```python
from build123d import *

# Parameters (mm, degrees)
F0_R     = 2
F1_DEPTH = 15
F2_W     = 15
F2_H     = 5
F3_DEPTH = 25.4


# Not quite as in the source:
# - a feature names something its author has since deleted; it is built from what else it names


with BuildPart() as f1:
    # F0 (on Top) → F1 (new body)
    with BuildSketch(Plane.XY):
        Polygon((-4, 0), (0, 0), (0, 15), (3, 15), (3, 0), (6, 0), (6, 25), (-4, 25), align=None)
        with Locations((1, 20)):
            Circle(F0_R, mode=Mode.SUBTRACT)
    extrude(amount=F1_DEPTH)

    # F2 (on face) → F3 (cut)
    with BuildSketch(Plane.YZ.offset(6)):
        with Locations((17.5, 7.5)):
            Rectangle(F2_W, F2_H)
    extrude(amount=-F3_DEPTH, mode=Mode.SUBTRACT)


solid = f1.part
```
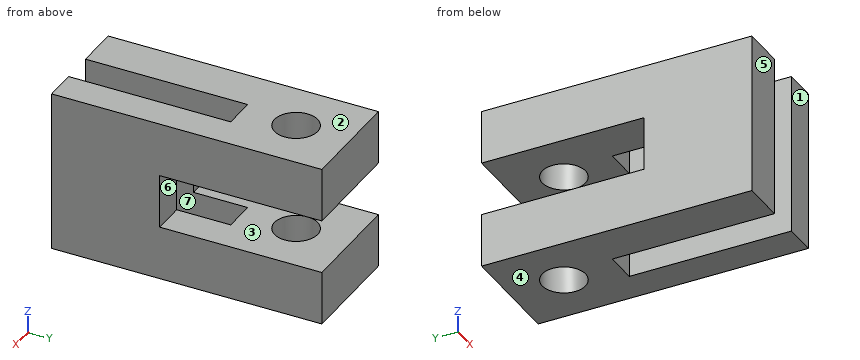
Read the model definition and answer for the solid it produces. Units are mm, in the model's axes. Face numbers are marked on the shaded views. A direction names the side the tool comes from. Give positions to 0.01 mm unless a question says otherwise; leave off trailing zeros. Order: outer loops, then holes, each group sorted by start corner. A loop starts at its lowest first (then second) coordinate and runs counter-clockwise, first axis right, second up.
(1) Find section C-C (z = 12). Give the vertices of the cut face in (x, y).
(2) Find section D-D (y = 20). Give the vertices of the cut face in (x, z).
(3) For a pull along Z with two mould halves and no side action, classify the marked faces 1, 2, 3 and 4 as released by +Z, released by -Z, zero draft, split by the parting line, or undercut.
(4) Find section B-B (y = 2.5). Give the vertices of the cut face in (x, z), plus the area to 3 significant figures.
(5) Find section A-A (x = 1). Give the vertices of the cut face in (y, z).
(6) Given pin 1 (0.9 mm diameter, centred on x = 1, z = 12.5, fed in from -Y); pin 2 (2 mm diameter, centred on x = -2, z = 8.5, fed in from +Y), each flat-ended and moving along its own axis, determine where each tip first touches the part or whether it passes through.
(7) For the marked faces 5, 6 and 7, determine the directions among +Z, -Z, +X, -X, +Y, -Y from which every point of the face is accessible in a straight line to the end or side of a thin tool.
(8) Straight lines are drawn through the part: L1, parallel to Z at x = 2.75, y = 16; L2, parallel to Y at x = 1, z = 11.1; L3, parallel to X at y = 20, z = 13.2. For each, find the intervals that lie inside material, in ascending order.
Result sheet:
1. outline: (-4, 0) - (0, 0) - (0, 15) - (3, 15) - (3, 0) - (6, 0) - (6, 25) - (-4, 25) - close; hole circle Ø4 at (1, 20)
2. outline: (-4, 0) - (-1, 0) - (-1, 5) - (-4, 5) - close; (-4, 10) - (-1, 10) - (-1, 15) - (-4, 15) - close; (3, 0) - (6, 0) - (6, 5) - (3, 5) - close; (3, 10) - (6, 10) - (6, 15) - (3, 15) - close
3. face 1: zero draft
3. face 2: released by +Z
3. face 3: undercut
3. face 4: released by -Z
4. outline: (-4, 0) - (0, 0) - (0, 15) - (-4, 15) - close; (3, 0) - (6, 0) - (6, 15) - (3, 15) - close
4. area: 105 mm2
5. outline: (15, 0) - (18, 0) - (18, 5) - (15, 5) - close; (15, 10) - (18, 10) - (18, 15) - (15, 15) - close; (22, 0) - (25, 0) - (25, 5) - (22, 5) - close; (22, 10) - (25, 10) - (25, 15) - (22, 15) - close
6. pin 1: stops at y = 15
6. pin 2: stops at y = 10
7. face 5: +Z, -Z, +X, -X, -Y
7. face 6: +X, -X, +Y
7. face 7: +Z, -Z, -Y
8. L1: z = 0 to 5, 10 to 15
8. L2: y = 15 to 18, 22 to 25
8. L3: x = -4 to -1, 3 to 6
